```python
from build123d import *

# Parameters (mm, degrees)
BOSS_EXTRUDE1_DEPTH      = 13
BOSS_EXTRUDE1_DEPTH_BACK = 3.35
SKETCH1_R                = 32
SKETCH1_R_2              = 22.25
SKETCH1_R_3              = 1.75


with BuildPart() as part:
    # Sketch1 → Boss-Extrude1 (new, two sides: drawn at the far end of the back side and taken through both)
    with BuildSketch(Plane(origin=(0, 0, 0), x_dir=(1, 0, 0), z_dir=(0, 1, 0)).offset(-BOSS_EXTRUDE1_DEPTH_BACK)):
        with Locations(Location((0, 0, 0), (0, 0, 270))):
            Circle(SKETCH1_R)
        with Locations(Location((0, 0, 0), (0, 0, 270))):
            Circle(SKETCH1_R_2, mode=Mode.SUBTRACT)
        with Locations(Location((27.75, 0, 0), (0, 0, 270))):
            Circle(SKETCH1_R_3, mode=Mode.SUBTRACT)
        with Locations(Location((-21.931253571, 17.002429733, 0), (0, 0, 270))):
            Circle(SKETCH1_R_3, mode=Mode.SUBTRACT)
        with Locations(Location((-21.931253571, -17.002429733, 0), (0, 0, 270))):
            Circle(SKETCH1_R_3, mode=Mode.SUBTRACT)
    extrude(amount=BOSS_EXTRUDE1_DEPTH + BOSS_EXTRUDE1_DEPTH_BACK)


solid = part.part
```
Read the model definition and answer for the solid it produces. Units are mm, in the model's axes. Coordinates: 2 decimals unless noted, no trailing zeros. Write each loop counter-clockwise with the first axis right and the second up, starting at its lowest first coordinate (ties: lowest second). Pieces come first, ordered by that corner, then holes. Notation, with made-up numbers: (64.25, 41.25) - (122.25, 41.25) arc R20 cw to (122.25, 62.25) - close; hole circle Ø8 at (-35.75, -27). An arc over 180 degrees is marked (long way). Answer as a JSON object with one key per item and string values. Group by question number.
1. A cutting plane is placed at C-C (z = 10). Determine the outline of the cut face in (x, y), plus the area to 3 significant figures.
2. Consider L1, parallel to X at y = 4.5, z = 0; L2, parallel to X at y = -0.25, z = -17; L3, parallel to Z at x = 13.5, y = 11. Determine where each line is inside the solid, lowest interval first. Write a range as [from, to].
3. A cutting plane is placed at D-D (y = 1). Determine the outline of the cut face in (x, z), plus the area to 3 significant figures.
4. A cutting plane is placed at A-A (z = 0). Determine the outline of the cut face in (x, y), plus the area to 3 significant figures.
5. Each of these flat-tipped pins is pushed along its axis until it touches: P1, Ø3, axis at x = -21.93, z = -17, coming from the +Y side; P2, Ø4, axis at y = 9, z = -7.5, coming from the +X side; P3, Ø2, axis at x = 3, y = 0.5, coming from the -Z side; P4, Ø2, axis at y = -0.5, z = -5.5, coming from the +X side. Where does it stop, or does it pass through?
6. A cutting plane is placed at B-B (x = 0). Determine the outline of the cut face in (y, z).
7. The mould has two halves that part along X. Classify faces 1 (the flat face through (-7, 13, -22)), 2 (the cylindrical face through (-31.24, 4.71, -6.94)), 3 (the cylindrical face through (-21.41, 4.71, -15.33)): +X half, -X half, draft (parallel to the pull), parting line (faces both ways), or undercut.
Worked out:
{
 "1": {"outline": "(-30.4, -3.35) - (-19.88, -3.35) - (-19.88, 13) - (-30.4, 13) - close; (19.88, -3.35) - (30.4, -3.35) - (30.4, 13) - (19.88, 13) - close", "area": "344 mm²"},
 "2": {"L1": "x = [-32, -22.25], [22.25, 26], [29.5, 32]", "L2": "x = [-27.11, -23.68], [-20.18, -14.35], [14.35, 27.11]", "L3": "z = [-29.01, -17.69], [17.69, 29.01]"},
 "3": {"outline": "circle Ø64 at (0, 0); hole circle Ø3.5 at (-21.93, -17); hole circle Ø3.5 at (-21.93, 17); hole circle Ø44.5 at (0, 0); hole circle Ø3.5 at (27.75, 0)", "area": "1,630 mm²"},
 "4": {"outline": "(-32, -3.35) - (-22.25, -3.35) - (-22.25, 13) - (-32, 13) - close; (22.25, -3.35) - (26, -3.35) - (26, 13) - (22.25, 13) - close; (29.5, -3.35) - (32, -3.35) - (32, 13) - (29.5, 13) - close", "area": "262 mm²"},
 "5": {"P1": "passes through", "P2": "stops at x = 31.52", "P3": "stops at z = -31.94", "P4": "stops at x = 31.68"},
 "6": {"outline": "(-3.35, -32) - (13, -32) - (13, -22.25) - (-3.35, -22.25) - close; (-3.35, 22.25) - (13, 22.25) - (13, 32) - (-3.35, 32) - close"},
 "7": {"face 1": "draft", "face 2": "parting line", "face 3": "undercut"}
}
